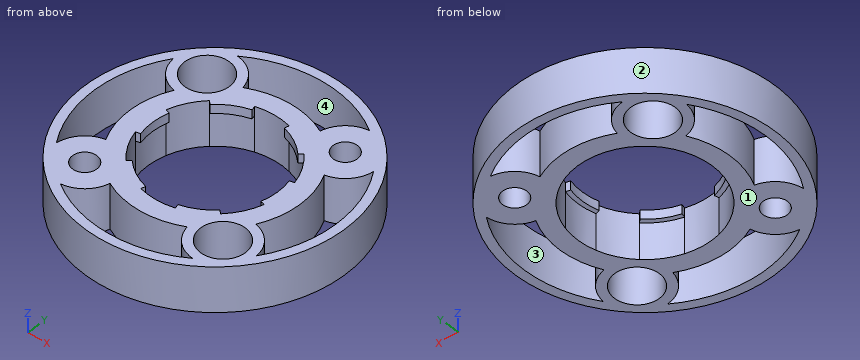
```python
from build123d import *

# Parameters (mm, degrees)
F0_R            = 23.01875
F0_R_2          = 2.15265
F0_R_3          = 3.96875
F0_R_4          = 11.1125
F1_DEPTH        = 7.9375
F3_DEPTH        = 7.9375
F4_COUNT        = 6
F4_ANGLE        = 300
F6_R            = 11.90625
F7_DEPTH        = 6.35
F9_DEPTH        = 7.9375
F9_COPIES_COUNT = 4


# Not quite as in the source:
# - a pattern or mirror of a feature is missing from the dataset's text; its kind, count and spacing are read off the source's solid


with BuildPart() as f1:
    # F0 (on Top) → F1 (new body)
    with BuildSketch(Plane.XY):
        Circle(F0_R)
        with Locations((-12.3478521665, -12.3478521665)):
            Circle(F0_R_2, mode=Mode.SUBTRACT)
        with Locations((12.3478521665, -12.3478521665)):
            Circle(F0_R_3, mode=Mode.SUBTRACT)
        with Locations((-12.3478521665, 12.3478521665)):
            Circle(F0_R_3, mode=Mode.SUBTRACT)
        Circle(F0_R_4, mode=Mode.SUBTRACT)
        with Locations((12.3478521665, 12.3478521665)):
            Circle(F0_R_2, mode=Mode.SUBTRACT)
    extrude(amount=F1_DEPTH)

    # F2 (on face) → F3 (cut, through all)
    with BuildSketch(Plane.XY.offset(7.9375)):
        with BuildLine():
            Line((-3.0815642558, 11.5005543693), (-2.8761266387, 10.7338507446))
            ThreePointArc((-2.8761266387, 10.7338507446), (0, 11.1125), (2.8761266387, 10.7338507446))
            Line((2.8761266387, 10.7338507446), (3.0815642558, 11.5005543693))
            ThreePointArc((3.0815642558, 11.5005543693), (0, 11.90625), (-3.0815642558, 11.5005543693))
        make_face()
    f3 = extrude(amount=-F3_DEPTH, mode=Mode.SUBTRACT)

    # F4: F3 ×6 about axis
    f4_axis = Axis((0, 0, 0), (0, 0, -1))
    for i in range(1, F4_COUNT):
        add(f3.rotate(f4_axis, i * F4_ANGLE / (F4_COUNT - 1)), mode=Mode.SUBTRACT)

    # F6 (on face) → F7 (cut, through all)
    with BuildSketch(Plane(origin=(0, 0, 0), x_dir=(1, 0, 0), z_dir=(0, 0, -1))):
        Circle(F6_R)
    extrude(amount=-F7_DEPTH, mode=Mode.SUBTRACT)

    # F8 (on face) → F9 (cut, through all)
    with BuildSketch(Plane(origin=(0, 0, 0), x_dir=(1, 0, 0), z_dir=(0, 0, -1))):
        with BuildLine():
            ThreePointArc((-13.4129757356, 6.8946489019), (-16.4630716815, 8.614638751), (-17.8787189274, 11.8173552911))
            ThreePointArc((-17.8787189274, 11.8173552911), (-21.43125, 0), (-17.8787189274, -11.8173552911))
            ThreePointArc((-17.8787189274, -11.8173552911), (-16.4630716815, -8.614638751), (-13.4129757356, -6.8946489019))
            ThreePointArc((-13.4129757356, -6.8946489019), (-15.08125, 0), (-13.4129757356, 6.8946489019))
        make_face()
    f9 = extrude(amount=-F9_DEPTH, mode=Mode.SUBTRACT)

    # F9_copies: F9 ×4 about axis
    f9_copies_axis = Axis((0, 0, 0), (0, 0, 1))
    for i in range(1, F9_COPIES_COUNT):
        add(f9.rotate(f9_copies_axis, i * 360 / F9_COPIES_COUNT), mode=Mode.SUBTRACT)


solid = f1.part
```
For this review, take the finished solid that the model builds, in its own axes (mm). Face numbers are marked on the shaded views. Round coordinates to 2 decimals unless told otherwise and drop trailing zeros. Write each loop counter-clockwise with the first axis right and the second up, starting at its lowest first coordinate (ties: lowest second). Pieces come first, ordered by that corner, then holes. Notation, with made-up numbers: (32, 31.25) -> (39, 31.25) arc R20 cw to (39, 39.25) -> close; hole circle Ø6 at (-12, 32.25). An arc over 180 degrees is marked (long way). One line per question, with ' | ' between items. Start each with the question number.
1) Wall thickness on line 1 along X through (y, z) = (-0.5, 4); line 2 along Y through (x, z) = (1.5, 1); line 3 along Y through (x, z) = (-13, 4.75): over which ranges is each line inside the solid? List them lowest first.
2) Add section D-D (z = 1). Count the separate pieces of the cut face and the enclosed holes in it, and give its area (3 significant figures).
3) For pin 1 Ø2 at (x, z) = (-14.5, 1) entering from -Y; pin 2 Ø3 at (x, z) = (-7.5, 6.5) entering from +Y; pin 3 Ø4 at (x, y) = (-12.35, -12.35) entering from -Z; pin 4 Ø1.5 at (y, z) = (5.5, 6) entering from +X, all flat-tipped, find the tip position at first contact; note any pin that passes through.
4) Add section A-A (y = 0). Write out the cut boundary in (x, z), and give its area (3 significant figures).
5) Add section B-B (x = 0). Write out the cut boundary in (y, z), and give its area (3 significant figures).
6) Add section C-C (x = 19). Write out the cut boundary in (y, z).
7) Mouldability with a two-part tool opening along X and no side actions: class the marked faces 1, 2, 3 and 4 as +X half, -X half, draft (parallel to the pull), parting line (faces both ways), or undercut.
Reported:
1) line 1: x = -23.01 to -21.43, -15.07 to -11.9, 11.9 to 15.07, 21.43 to 23.01 | line 2: y = -22.97 to -21.38, -15.01 to -11.81, 11.81 to 15.01, 21.38 to 22.97 | line 3: y = -19 to -14.4, -10.3 to 8.43, 16.26 to 19
2) separate pieces: 1 | enclosed holes: 9 | area: 631 mm²
3) pin 1: stops at y = -18.64 | pin 2: stops at y = 22.22 | pin 3: passes through | pin 4: stops at x = 22.52
4) outline: (-23.02, 0) -> (-21.43, 0) -> (-21.43, 7.94) -> (-23.02, 7.94) -> close; (-15.08, 0) -> (-11.91, 0) -> (-11.91, 6.35) -> (-11.11, 6.35) -> (-11.11, 7.94) -> (-15.08, 7.94) -> close; (11.11, 6.35) -> (11.91, 6.35) -> (11.91, 0) -> (15.08, 0) -> (15.08, 7.94) -> (11.11, 7.94) -> close; (21.43, 0) -> (23.02, 0) -> (23.02, 7.94) -> (21.43, 7.94) -> close | area: 78.1 mm²
5) outline: (-23.02, 0) -> (-21.43, 0) -> (-21.43, 7.94) -> (-23.02, 7.94) -> close; (-15.08, 0) -> (-11.91, 0) -> (-11.91, 7.94) -> (-15.08, 7.94) -> close; (11.91, 0) -> (15.08, 0) -> (15.08, 7.94) -> (11.91, 7.94) -> close; (21.43, 0) -> (23.02, 0) -> (23.02, 7.94) -> (21.43, 7.94) -> close | area: 75.6 mm²
6) outline: (-12.99, 0) -> (-9.91, 0) -> (-9.91, 7.94) -> (-12.99, 7.94) -> close; (9.91, 0) -> (12.99, 0) -> (12.99, 7.94) -> (9.91, 7.94) -> close
7) face 1: draft | face 2: parting line | face 3: undercut | face 4: undercut
